```python
from build123d import *

# Parameters (mm, degrees)
SKETCH1_W            = 25
SKETCH1_H            = 45
SKETCH1_W_2          = 21
SKETCH1_H_2          = 41
BOSS_EXTRUDE1_DEPTH  = 186.9
M4_CLEARANCE_HOLE1_D = 4.5


with BuildPart() as part:
    # Sketch1 → Boss-Extrude1 (new body)
    with BuildSketch(Plane.XY.offset(40)):
        Rectangle(SKETCH1_W, SKETCH1_H)
        Rectangle(SKETCH1_W_2, SKETCH1_H_2, mode=Mode.SUBTRACT)
    extrude(amount=BOSS_EXTRUDE1_DEPTH)

    # M4 Clearance Hole1 (through all)
    with Locations(Plane(origin=(12.5, 0, 0), x_dir=(0, 0, -1), z_dir=(1, 0, 0))):
        with Locations((-45, -12.5), (-45, 12.5), (-221.9, 12.5), (-221.9, -12.5)):
            Hole(M4_CLEARANCE_HOLE1_D / 2)


solid = part.part
```
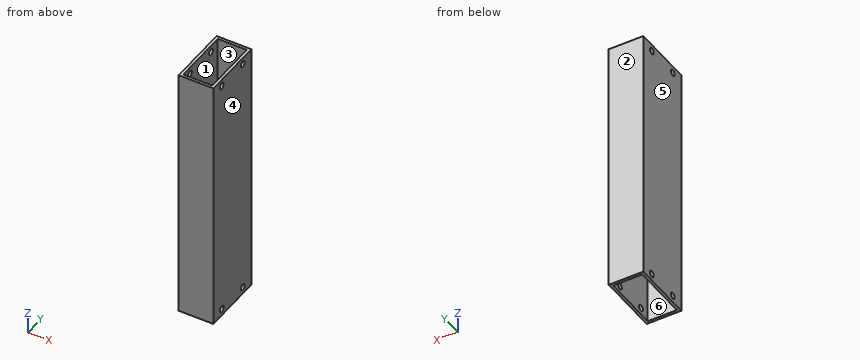
For this review, take the finished solid that the model builds, in its own axes (mm). Face numbers are marked on the shaded views. A direction names the side the tool comes from. Give positions to 0.01 mm unless a question says otherwise; leave off trailing zeros. Write each loop counter-clockwise with the first axis right and the second up, starting at its lowest first coordinate (ties: lowest second). Pieces come first, ordered by that corner, then holes. Notation, with made-up numbers: M 42.5,-26.75 L 63.5,-26.75 A24 cw 63.5,3.25 Z; hole C 55.5,17 d1. An arc over 180 degrees is marked long. One line per item, written item: value.
1) For the marked faces 1 and 2, list the 3-axis set-ups (+Z, -Z, +X, -X, +Y, -Y) from which the entire face can be reached by the end or side of a thin tool; tool diameter is ignored.
Results are:
face 1: +Z, -Z
face 2: +Z, -Z, +X, -X, +Y
2) For line 1 (Y direction, x = 11.15, z = 45); line 2 (X direction, y = -13, z = 171); line 3 (Y direction, x = 0, z = 173), list the stretches that pass through material, from the lowest coordinate up. Write a range as from..to.
Results are:
line 1: y = -22.5..-14.75, -10.25..10.25, 14.75..22.5
line 2: x = -12.5..-10.5, 10.5..12.5
line 3: y = -22.5..-20.5, 20.5..22.5
3) Take a section at A-A, the plane y = 12.5. Write out the cut boundary in (x, z).
Results are:
outline: M -12.5,40 L -10.5,40 L -10.5,42.75 L -12.5,42.75 Z; M -12.5,47.25 L -10.5,47.25 L -10.5,219.65 L -12.5,219.65 Z; M -12.5,224.15 L -10.5,224.15 L -10.5,226.9 L -12.5,226.9 Z; M 10.5,40 L 12.5,40 L 12.5,42.75 L 10.5,42.75 Z; M 10.5,47.25 L 12.5,47.25 L 12.5,219.65 L 10.5,219.65 Z; M 10.5,224.15 L 12.5,224.15 L 12.5,226.9 L 10.5,226.9 Z
4) The part is to be moulded in two halves that separate along X. For the marked faces 3, 4, 5 and 6, say which applies: +X half, -X half, draft (parallel to the pull), parting line (faces both ways), or undercut.
Results are:
face 3: undercut
face 4: +X half
face 5: -X half
face 6: undercut
5) For P1, Ø4, axis at y = -12.5, z = 45, coming from the -X side, flat-tipped, find the tip position at first contact; note if it passes through.
Results are:
P1: passes through
6) Take a section at B-B, the plane z = 221.9. Write out the cut boundary in (x, y).
Results are:
outline: M -12.5,-22.5 L 12.5,-22.5 L 12.5,-14.75 L 10.5,-14.75 L 10.5,-20.5 L -10.5,-20.5 L -10.5,-14.75 L -12.5,-14.75 Z; M -12.5,-10.25 L -10.5,-10.25 L -10.5,10.25 L -12.5,10.25 Z; M -12.5,14.75 L -10.5,14.75 L -10.5,20.5 L 10.5,20.5 L 10.5,14.75 L 12.5,14.75 L 12.5,22.5 L -12.5,22.5 Z; M 10.5,-10.25 L 12.5,-10.25 L 12.5,10.25 L 10.5,10.25 Z
7) Take a section at C-C, the plane y = 2. Write out the cut boundary in (x, z).
Results are:
outline: M -12.5,40 L -10.5,40 L -10.5,226.9 L -12.5,226.9 Z; M 10.5,40 L 12.5,40 L 12.5,226.9 L 10.5,226.9 Z
8) Take a section at D-D, the plane x = -7.75. Write out the cut boundary in (y, z).
Results are:
outline: M -22.5,40 L -20.5,40 L -20.5,226.9 L -22.5,226.9 Z; M 20.5,40 L 22.5,40 L 22.5,226.9 L 20.5,226.9 Z
